Work out the finished part from the listing and answer in its coordinate system (mm). A direction names the side the tool comes from. Give positions to 0.01 mm unless a question says otherwise; leave off trailing zeros. Write each loop counter-clockwise with the first axis right and the second up, starting at its lowest first coordinate (ties: lowest second). Pieces come first, ordered by that corner, then holes.
1) Given pin 1 Ø9 at (y, z) = (-2, -10.5) entering from +X; pin 2 Ø9 at (y, z) = (-1, -22) entering from -X; pin 3 Ø8 at (x, y) = (-41, 69) entering from -Z, each flat-ended and moving along its own axis, determine where each tip first touches the part or whether it passes through.
2) Find section D-D (x = -118). Determine the outline of the cut face in (y, z).
3) Find section A-A (y = -70.5). Determine the outline of the cut face in (x, z).
4) A tool of negligible diameter and unlimited length cuts with its end or side. For faces 1 (the face through (-25, 0, -15)), 2 (the face through (-35, 0, -20)), 3 (the face through (35, 0, -20)), 4 (the face through (-240, 4, 152)), 5 (the face through (0, -20, -34)), from which of +Z, -Z, +X, -X, +Y, -Y can it reach the whole face along a straight path? Write none if from no direction.
5) Straight lines are drawn through the part: probe 1 along X at (y, z) = (8, 168); probe 2 along Z at (x, y) = (24.5, 12.5); probe 3 along Z at (x, y) = (-161, -89). For each, find the intervals that lie inside material, in ascending order.
6) Find section C-C (z = 67.5). Determine the outline of the cut face in (x, y), plus the area to 3 significant figures.
7) Find section B-B (y = -14.5). Determine the outline of the cut face in (x, z), plus the area to 3 significant figures.
```python
from build123d import *

# Parameters (mm, degrees)
SKETCH1_W                = 500
SKETCH1_H                = 200
BOSS_EXTRUDE1_DEPTH      = 300
BOSS_EXTRUDE2_DEPTH      = 20
BOSS_EXTRUDE2_DEPTH_BACK = 20
SHELL1_START             = -240
SHELL1_OUTLINE_W         = 190
SHELL1_OUTLINE_H         = 280
SHELL1_DEPTH             = 480


# Read off the part's stored shape, not the designer's step: Shell1
with BuildPart() as part:
    # Sketch1 → Boss-Extrude1 (new body)
    with BuildSketch(Plane.XY):
        Rectangle(SKETCH1_W, SKETCH1_H)
    extrude(amount=BOSS_EXTRUDE1_DEPTH)

    # Sketch2 → Boss-Extrude2 (add, two sides: drawn at the far end of the back side and taken through both)
    with BuildSketch(Plane(origin=(0, 0, 0), x_dir=(1, 0, 0), z_dir=(0, 1, 0)).offset(-BOSS_EXTRUDE2_DEPTH_BACK)):
        Polygon((25, 0), (25, 30), (-25, 30), (-25, 0), (-35, 0), (-35, 40), (35, 40), (35, 0), align=None)
    extrude(amount=BOSS_EXTRUDE2_DEPTH + BOSS_EXTRUDE2_DEPTH_BACK)

    # Shell1 outline → Shell1 (cut)
    with BuildSketch(Plane.YZ.offset(SHELL1_START)):
        with Locations((5, 150)):
            Rectangle(SHELL1_OUTLINE_W, SHELL1_OUTLINE_H)
    extrude(amount=SHELL1_DEPTH, mode=Mode.SUBTRACT)


solid = part.part
```
Results:
1. pin 1: stops at x = 35
1. pin 2: stops at x = -35
1. pin 3: stops at z = 0
2. outline: (-100, 0) - (100, 0) - (100, 10) - (-90, 10) - (-90, 290) - (100, 290) - (100, 300) - (-100, 300) - close
3. outline: (-250, 0) - (250, 0) - (250, 300) - (-250, 300) - close; hole (-240, 10) - (240, 10) - (240, 290) - (-240, 290) - close
4. face 1: +Y, -Y
4. face 2: -Z, -X, +Y, -Y
4. face 3: -Z, +X, +Y, -Y
4. face 4: +Y
4. face 5: -Z, +X, -X, -Y
5. probe 1: x = -250 to -240, 240 to 250
5. probe 2: z = -40 to -30, 0 to 10, 290 to 300
5. probe 3: z = 0 to 10, 290 to 300
6. outline: (-250, -100) - (250, -100) - (250, 100) - (240, 100) - (240, -90) - (-240, -90) - (-240, 100) - (-250, 100) - close
6. area: 8,800 mm2
7. outline: (-250, 0) - (-35, 0) - (-35, -40) - (35, -40) - (35, 0) - (250, 0) - (250, 300) - (-250, 300) - close; hole (-240, 10) - (240, 10) - (240, 290) - (-240, 290) - close; hole (-25, -30) - (25, -30) - (25, 0) - (-25, 0) - close
7. area: 16,900 mm2
